```python
from build123d import *

# Parameters (mm, degrees)
SKETCH1_W           = 190.5
SKETCH1_H           = 101.6
BOSS_EXTRUDE1_DEPTH = 6.35
SKETCH2_W           = 8.89
SKETCH2_H           = 76.2
HOLE_DEPTH          = 6.35
SKETCH3_W           = 38.1
SKETCH3_H           = 6.35
TAB1_DEPTH          = 6.35
SKETCH4_W           = 38.1
SKETCH4_H           = 6.35
TAB2_DEPTH          = 6.35


with BuildPart() as part:
    # Sketch1 → Boss-Extrude1 (new body)
    with BuildSketch(Plane(origin=(0, 0, 0), x_dir=(1, 0, 0), z_dir=(0, 1, 0))):
        Rectangle(SKETCH1_W, SKETCH1_H)
    extrude(amount=BOSS_EXTRUDE1_DEPTH)

    # Sketch2 → hole (cut)
    with BuildSketch(Plane(origin=(0, 6.35, 0), x_dir=(1, 0, 0), z_dir=(0, 1, 0))):
        with Locations((-48.768, 0)):
            Rectangle(SKETCH2_W, SKETCH2_H)
        with Locations((-13.208, 0)):
            Rectangle(SKETCH2_W, SKETCH2_H)
        with Locations((22.352, 0)):
            Rectangle(SKETCH2_W, SKETCH2_H)
        with Locations((57.912, 0)):
            Rectangle(SKETCH2_W, SKETCH2_H)
    extrude(amount=-HOLE_DEPTH, mode=Mode.SUBTRACT)

    # Sketch3 → tab1 (add)
    with BuildSketch(Plane.ZY.offset(95.25)):
        with Locations((0, 3.175)):
            Rectangle(SKETCH3_W, SKETCH3_H)
    extrude(amount=TAB1_DEPTH)

    # Sketch4 → tab2 (add)
    with BuildSketch(Plane(origin=(95.25, 0, 0), x_dir=(0, 0, -1), z_dir=(1, 0, 0))):
        with Locations((0, 3.175)):
            Rectangle(SKETCH4_W, SKETCH4_H)
    extrude(amount=TAB2_DEPTH)


solid = part.part
```
Here's how the part is built. I have some questions about the finished solid (model axes, mm). A direction names the side the tool comes from. Round coordinates to 2 decimals unless told otherwise and drop trailing zeros. Write each loop counter-clockwise with the first axis right and the second up, starting at its lowest first coordinate (ties: lowest second). Pieces come first, ordered by that corner, then holes. Notation, with made-up numbers: M 73,-29 L 79,-29 A35 cw 79,10 Z; hole C -14.5,35 d10. An arc over 180 degrees is marked long. Answer as CSV lines item,"result". Start each with the question number.
1. I'm going to push flat-ended pins straight in: pin 1 Ø1.5 at (y, z) = (1.5, -28.5) entering from +X; pin 2 Ø1 at (y, z) = (1, 28) entering from -X; pin 3 Ø3 at (x, y) = (98.5, 4) entering from -Z. Where does each tip first touch, or does it pass through?
2. Suppose I cut it at D-D on z = 24. Write out the boundary of the cut face in (x, y), then the cut area to 3 significant figures.
3. Suppose I cut it at C-C on y = 2.5. Write out the boundary of the cut face in (x, z), then the cut area to 3 significant figures.
4. I need wall thicknesses on probe 1 along X at (y, z) = (2, 2); probe 2 along X at (y, z) = (4.25, -36.5); probe 3 along Z at (x, y) = (-14, 2.5). Which ranges of each line are inside material? Lowest first, please.
5. Thinking about a two-plate mould opening in X: for faces 6 (the flat face through (95.25, 3, 35)), 7 (the flat face through (17.907, 3, 1)), 8 (the flat face through (98, 3, -19.05)), which applies, released by +X, released by -X, zero draft, split by the parting line, or undercut?
6. Suppose I cut it at A-A on z = -9. Write out the boundary of the cut face in (x, y).
7. Suppose I cut it at B-B on x = -13.5. Write out the boundary of the cut face in (y, z).
8. On a 3-axis mill with a long thin cutter (end or side, diameter ignored), from which of +Z, -Z, +X, -X, +Y, -Y can I reach the whole of each face in a straight line? I mean faces 1 (the flat face through (-1, 3, -50.8)), 2 (the flat face through (-1, 6.35, -1)), 3 (the flat face through (62.357, 3, 1)), 4 (the flat face through (-98, 3, -19.05)), 5 (the flat face through (-95.25, 3, 35)). Say none if no direction works.
Check result:
1,pin 1,"stops at x = 95.25"
1,pin 2,"stops at x = -95.25"
1,pin 3,"stops at z = -19.05"
2,outline,"M -95.25,0 L -53.21,0 L -53.21,6.35 L -95.25,6.35 Z; M -44.32,0 L -17.65,0 L -17.65,6.35 L -44.32,6.35 Z; M -8.76,0 L 17.91,0 L 17.91,6.35 L -8.76,6.35 Z; M 26.8,0 L 53.47,0 L 53.47,6.35 L 26.8,6.35 Z; M 62.36,0 L 95.25,0 L 95.25,6.35 L 62.36,6.35 Z"
2,area,"984 mm2"
3,outline,"M -101.6,-19.05 L -95.25,-19.05 L -95.25,-50.8 L 95.25,-50.8 L 95.25,-19.05 L 101.6,-19.05 L 101.6,19.05 L 95.25,19.05 L 95.25,50.8 L -95.25,50.8 L -95.25,19.05 L -101.6,19.05 Z; hole M -53.21,-38.1 L -44.32,-38.1 L -44.32,38.1 L -53.21,38.1 Z; hole M -17.65,-38.1 L -8.76,-38.1 L -8.76,38.1 L -17.65,38.1 Z; hole M 17.91,-38.1 L 26.8,-38.1 L 26.8,38.1 L 17.91,38.1 Z; hole M 53.47,-38.1 L 62.36,-38.1 L 62.36,38.1 L 53.47,38.1 Z"
3,area,"17,100 mm2"
4,probe 1,"x = -101.6 to -53.21, -44.32 to -17.65, -8.76 to 17.91, 26.8 to 53.47, 62.36 to 101.6"
4,probe 2,"x = -95.25 to -53.21, -44.32 to -17.65, -8.76 to 17.91, 26.8 to 53.47, 62.36 to 95.25"
4,probe 3,"z = -50.8 to -38.1, 38.1 to 50.8"
5,face 6,"released by +X"
5,face 7,"undercut"
5,face 8,"zero draft"
6,outline,"M -101.6,0 L -53.21,0 L -53.21,6.35 L -101.6,6.35 Z; M -44.32,0 L -17.65,0 L -17.65,6.35 L -44.32,6.35 Z; M -8.76,0 L 17.91,0 L 17.91,6.35 L -8.76,6.35 Z; M 26.8,0 L 53.47,0 L 53.47,6.35 L 26.8,6.35 Z; M 62.36,0 L 101.6,0 L 101.6,6.35 L 62.36,6.35 Z"
7,outline,"M 0,-50.8 L 6.35,-50.8 L 6.35,-38.1 L 0,-38.1 Z; M 0,38.1 L 6.35,38.1 L 6.35,50.8 L 0,50.8 Z"
8,face 1,"-Z, +X, -X, +Y, -Y"
8,face 2,"+Z, -Z, +X, -X, +Y"
8,face 3,"+Y, -Y"
8,face 4,"-Z, -X, +Y, -Y"
8,face 5,"+Z, -X, +Y, -Y"
